CAD build for the part. Positions are in the model's coordinates, mm. Face numbers are marked on the shaded views. A direction names the side the tool comes from. Coordinates: 2 decimals unless noted, no trailing zeros. Loops run counter-clockwise (first coordinate to the right, second up) from the corner with the lowest first, then second, coordinate; pieces in that order, holes last. Notation, with made-up numbers: (60, 43.5) - (85, 43.5) arc R27 cw to (85, 82.5) - close; hole circle Ø5 at (61, 39). An arc over 180 degrees is marked (long way). Put each result on its own line as item: value.
```python
from build123d import *

# Parameters (mm, degrees)
F1_DEPTH = 25.4


with BuildPart() as f1:
    # F0 (on Top) → F1 (new body)
    with BuildSketch(Plane.XY):
        with BuildLine():
            ThreePointArc((0.0883997278, 32.8236170641), (-13.058763384, 37.4885196208), (-20.2230135431, 49.4585962042))
            ThreePointArc((-20.2230135431, 49.4585962042), (-53.4333511512, 0), (-20.2230135431, -49.4585962042))
            ThreePointArc((-20.2230135431, -49.4585962042), (-13.0929285798, -37.5165620637), (0, -32.8234274819))
            Line((0, -32.8234274819), (42.1633208321, -32.8234274819))
            ThreePointArc((42.1633208321, -32.8234274819), (50.5373651023, -17.3521682727), (53.4333511512, 0))
            ThreePointArc((53.4333511512, 0), (50.5373260912, 17.3522818904), (42.1631732449, 32.8236170641))
            Line((42.1631732449, 32.8236170641), (0.0883997278, 32.8236170641))
        make_face()
        with BuildLine():
            ThreePointArc((0, -32.8234274819), (-13.0929285798, -37.5165620637), (-20.2230135431, -49.4585962042))
            ThreePointArc((-20.2230135431, -49.4585962042), (-10.3049618346, -52.4302467745), (0, -53.4333511512))
            ThreePointArc((0, -53.4333511512), (10.3049618346, -52.4302467745), (20.2230135431, -49.4585962042))
            ThreePointArc((20.2230135431, -49.4585962042), (13.0929285798, -37.5165620637), (0, -32.8234274819))
        make_face()
        with BuildLine():
            ThreePointArc((0, -32.8234274819), (13.0929285798, -37.5165620637), (20.2230135431, -49.4585962042))
            ThreePointArc((20.2230135431, -49.4585962042), (32.2830588513, -42.5784819651), (42.1633208321, -32.8234274819))
            Line((42.1633208321, -32.8234274819), (0, -32.8234274819))
        make_face()
        with BuildLine():
            Line((0, -53.4333511512), (20.6099236693, -53.4333511512))
            ThreePointArc((20.6099236693, -53.4333511512), (20.5129680829, -51.436580237), (20.2230135431, -49.4585962042))
            ThreePointArc((20.2230135431, -49.4585962042), (10.3049618346, -52.4302467745), (0, -53.4333511512))
        make_face()
        with BuildLine():
            Line((20.6099236693, -53.4333511512), (51.2570339651, -53.4333511512))
            ThreePointArc((51.2570339651, -53.4333511512), (59.7096740135, -43.7854013954), (66.3703936593, -32.8234274819))
            Line((66.3703936593, -32.8234274819), (42.1633208321, -32.8234274819))
            ThreePointArc((42.1633208321, -32.8234274819), (32.2830588513, -42.5784819651), (20.2230135431, -49.4585962042))
            ThreePointArc((20.2230135431, -49.4585962042), (20.5129680829, -51.436580237), (20.6099236693, -53.4333511512))
        make_face()
        with BuildLine():
            ThreePointArc((102.2053944331, -32.8234274819), (87.6319776468, -38.8599343649), (81.5954707638, -53.4333511512))
            Line((81.5954707638, -53.4333511512), (102.2053944331, -53.4333511512))
            Line((102.2053944331, -53.4333511512), (102.2053944331, -32.8234274819))
        make_face()
        with BuildLine():
            ThreePointArc((20.6099236693, 53.4333511512), (14.5734167863, 68.0067679375), (0, 74.0432748205))
            ThreePointArc((0, 74.0432748205), (-15.9167890876, 66.526279731), (-20.2230135431, 49.4585962042))
            ThreePointArc((-20.2230135431, 49.4585962042), (-10.3049618346, 52.4302467745), (0, 53.4333511512))
            Line((0, 53.4333511512), (20.6099236693, 53.4333511512))
        make_face()
        with BuildLine():
            ThreePointArc((51.2570339651, 53.4333511512), (27.6226921414, 68.6978414873), (0, 74.0432748205))
            ThreePointArc((0, 74.0432748205), (14.5734167863, 68.0067679375), (20.6099236693, 53.4333511512))
            Line((20.6099236693, 53.4333511512), (51.2570339651, 53.4333511512))
        make_face()
        with BuildLine():
            ThreePointArc((81.5954707638, -53.4333511512), (87.6319776468, -68.0067679375), (102.2053944331, -74.0432748205))
            Line((102.2053944331, -74.0432748205), (102.2053944331, -53.4333511512))
            Line((102.2053944331, -53.4333511512), (81.5954707638, -53.4333511512))
        make_face()
        with BuildLine():
            Line((102.2053944331, 74.0432748205), (0, 74.0432748205))
            ThreePointArc((0, 74.0432748205), (27.6226921414, 68.6978414873), (51.2570339651, 53.4333511512))
            Line((51.2570339651, 53.4333511512), (81.5954707638, 53.4333511512))
            ThreePointArc((81.5954707638, 53.4333511512), (87.6319776468, 68.0067679375), (102.2053944331, 74.0432748205))
        make_face()
        with BuildLine():
            ThreePointArc((-20.2230135431, -49.4585962042), (-15.9167890876, -66.526279731), (0, -74.0432748205))
            ThreePointArc((0, -74.0432748205), (14.5734167863, -68.0067679375), (20.6099236693, -53.4333511512))
            Line((20.6099236693, -53.4333511512), (0, -53.4333511512))
            ThreePointArc((0, -53.4333511512), (-10.3049618346, -52.4302467745), (-20.2230135431, -49.4585962042))
        make_face()
        with BuildLine():
            ThreePointArc((122.8153181024, 53.4333511512), (116.7788112194, 68.0067679375), (102.2053944331, 74.0432748205))
            Line((102.2053944331, 74.0432748205), (102.2053944331, 53.4333511512))
            Line((102.2053944331, 53.4333511512), (102.2053944331, 32.8236170641))
            Line((102.2053944331, 32.8236170641), (102.2053944331, 32.8234274819))
            ThreePointArc((102.2053944331, 32.8234274819), (116.7788112194, 38.8599343649), (122.8153181024, 53.4333511512))
        make_face()
        with BuildLine():
            Line((102.2053944331, 53.4333511512), (102.2053944331, 74.0432748205))
            ThreePointArc((102.2053944331, 74.0432748205), (87.6319776468, 68.0067679375), (81.5954707638, 53.4333511512))
            Line((81.5954707638, 53.4333511512), (102.2053944331, 53.4333511512))
        make_face()
        with BuildLine():
            ThreePointArc((20.6099236693, -53.4333511512), (14.5734167863, -68.0067679375), (0, -74.0432748205))
            ThreePointArc((0, -74.0432748205), (27.6226921414, -68.6978414873), (51.2570339651, -53.4333511512))
            Line((51.2570339651, -53.4333511512), (20.6099236693, -53.4333511512))
        make_face()
        with BuildLine():
            ThreePointArc((51.2570339651, -53.4333511512), (27.6226921414, -68.6978414873), (0, -74.0432748205))
            Line((0, -74.0432748205), (102.2053944331, -74.0432748205))
            ThreePointArc((102.2053944331, -74.0432748205), (87.6319776468, -68.0067679375), (81.5954707638, -53.4333511512))
            Line((81.5954707638, -53.4333511512), (51.2570339651, -53.4333511512))
        make_face()
        with BuildLine():
            ThreePointArc((-20.2230135431, 49.4585962042), (-15.9167890876, 66.526279731), (0, 74.0432748205))
            ThreePointArc((0, 74.0432748205), (-74.0432748205, 0), (0, -74.0432748205))
            ThreePointArc((0, -74.0432748205), (-15.9167890876, -66.526279731), (-20.2230135431, -49.4585962042))
            ThreePointArc((-20.2230135431, -49.4585962042), (-53.4333511512, 0), (-20.2230135431, 49.4585962042))
        make_face()
        with BuildLine():
            ThreePointArc((66.3703936593, -32.8234274819), (59.7096740135, -43.7854013954), (51.2570339651, -53.4333511512))
            Line((51.2570339651, -53.4333511512), (81.5954707638, -53.4333511512))
            ThreePointArc((81.5954707638, -53.4333511512), (87.6319776468, -38.8599343649), (102.2053944331, -32.8234274819))
            Line((102.2053944331, -32.8234274819), (66.3703936593, -32.8234274819))
        make_face()
        with BuildLine():
            Line((102.2053944331, 32.8236170641), (102.1169947054, 32.8236170641))
            ThreePointArc((102.1169947054, 32.8236170641), (102.1611944676, 32.8234748775), (102.2053944331, 32.8234274819))
            Line((102.2053944331, 32.8234274819), (102.2053944331, 32.8236170641))
        make_face()
        with BuildLine():
            Line((102.2053944331, -53.4333511512), (102.2053944331, -74.0432748205))
            ThreePointArc((102.2053944331, -74.0432748205), (116.7788112194, -68.0067679375), (122.8153181024, -53.4333511512))
            ThreePointArc((122.8153181024, -53.4333511512), (116.7788112194, -38.8599343649), (102.2053944331, -32.8234274819))
            Line((102.2053944331, -32.8234274819), (102.2053944331, -53.4333511512))
        make_face()
        with BuildLine():
            Line((102.2053944331, 53.4333511512), (81.5954707638, 53.4333511512))
            ThreePointArc((81.5954707638, 53.4333511512), (87.6007570653, 38.891221974), (102.1169947054, 32.8236170641))
            Line((102.1169947054, 32.8236170641), (102.2053944331, 32.8236170641))
            Line((102.2053944331, 32.8236170641), (102.2053944331, 53.4333511512))
        make_face()
        with BuildLine():
            Line((81.5954707638, 53.4333511512), (51.2570339651, 53.4333511512))
            ThreePointArc((51.2570339651, 53.4333511512), (59.7096114785, 43.7854866736), (66.3702999012, 32.8236170641))
            Line((66.3702999012, 32.8236170641), (102.1169947054, 32.8236170641))
            ThreePointArc((102.1169947054, 32.8236170641), (87.6007570653, 38.891221974), (81.5954707638, 53.4333511512))
        make_face()
        with BuildLine():
            ThreePointArc((66.3702999012, 32.8236170641), (59.7096114785, 43.7854866736), (51.2570339651, 53.4333511512))
            Line((51.2570339651, 53.4333511512), (20.6099236693, 53.4333511512))
            ThreePointArc((20.6099236693, 53.4333511512), (20.5129680829, 51.436580237), (20.2230135431, 49.4585962042))
            ThreePointArc((20.2230135431, 49.4585962042), (32.2829631266, 42.5785545435), (42.1631732449, 32.8236170641))
            Line((42.1631732449, 32.8236170641), (66.3702999012, 32.8236170641))
        make_face()
        with BuildLine():
            ThreePointArc((20.2230135431, 49.4585962042), (20.5129680829, 51.436580237), (20.6099236693, 53.4333511512))
            Line((20.6099236693, 53.4333511512), (0, 53.4333511512))
            ThreePointArc((0, 53.4333511512), (10.3049618346, 52.4302467745), (20.2230135431, 49.4585962042))
        make_face()
        with BuildLine():
            ThreePointArc((0, 53.4333511512), (-10.3049618346, 52.4302467745), (-20.2230135431, 49.4585962042))
            ThreePointArc((-20.2230135431, 49.4585962042), (-13.058763384, 37.4885196208), (0.0883997278, 32.8236170641))
            ThreePointArc((0.0883997278, 32.8236170641), (13.1270335572, 37.5446777126), (20.2230135431, 49.4585962042))
            ThreePointArc((20.2230135431, 49.4585962042), (10.3049618346, 52.4302467745), (0, 53.4333511512))
        make_face()
        with BuildLine():
            ThreePointArc((74.0432748205, 0), (72.0995176879, 16.8542604501), (66.3702999012, 32.8236170641))
            Line((66.3702999012, 32.8236170641), (42.1631732449, 32.8236170641))
            ThreePointArc((42.1631732449, 32.8236170641), (50.5373260912, 17.3522818904), (53.4333511512, 0))
            Line((53.4333511512, 0), (74.0432748205, 0))
        make_face()
        with BuildLine():
            Line((42.1633208321, -32.8234274819), (66.3703936593, -32.8234274819))
            ThreePointArc((66.3703936593, -32.8234274819), (72.0995417593, -16.8541574765), (74.0432748205, 0))
            Line((74.0432748205, 0), (53.4333511512, 0))
            ThreePointArc((53.4333511512, 0), (50.5373651023, -17.3521682727), (42.1633208321, -32.8234274819))
        make_face()
        with BuildLine():
            ThreePointArc((42.1631732449, 32.8236170641), (32.2829631266, 42.5785545435), (20.2230135431, 49.4585962042))
            ThreePointArc((20.2230135431, 49.4585962042), (13.1270335572, 37.5446777126), (0.0883997278, 32.8236170641))
            Line((0.0883997278, 32.8236170641), (42.1631732449, 32.8236170641))
        make_face()
    extrude(amount=F1_DEPTH)


solid = f1.part
```
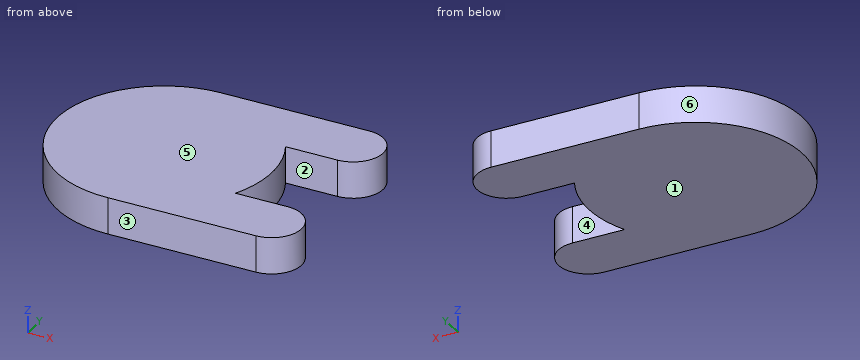
Q1. Slice it at D-D, the plane x = -34. Give the cut face in (y, z), then the cut area to 3 significant figures.
Determined:
outline: (-65.78, 0) - (65.78, 0) - (65.78, 25.4) - (-65.78, 25.4) - close
area: 3,340 mm2
Q2. Slice it at A-A, the plane z = 2. Give the cut face in (x, y).
Determined:
outline: (0, -74.04) - (102.21, -74.04) arc R20.61 ccw to (102.21, -32.82) - (66.37, -32.82) arc R74.04 ccw to (66.37, 32.82) - (102.12, 32.82) arc R20.61 ccw to (102.21, 32.82) arc R20.61 ccw to (102.21, 74.04) - (0, 74.04) arc R74.04 ccw to start
Q3. Slice it at B-B, the plane x = 71. Give the cut face in (y, z).
Determined:
outline: (-74.04, 0) - (-32.82, 0) - (-32.82, 25.4) - (-74.04, 25.4) - close; (-21.01, 0) - (21.01, 0) - (21.01, 25.4) - (-21.01, 25.4) - close; (32.82, 0) - (74.04, 0) - (74.04, 25.4) - (32.82, 25.4) - close
Q4. Slice it at C-C, the plane y = 0. Give the cut face in (x, z).
Determined:
outline: (-74.04, 0) - (74.04, 0) - (74.04, 25.4) - (-74.04, 25.4) - close
Q5. Wall check: L1, parallel to Y at x = 96, z = 20; L2, parallel to X at y = -4, z = 8.5; L3, parallel to X at y = -15, z = 14.5. Give the ranges that are in metal, low to high. Write a range as from..to.
Determined:
L1: -74.04..-32.82, 32.82..74.04
L2: -73.94..73.94
L3: -72.51..72.51
Q6. Pin check, flat tips, straight feed: pin 1 Ø6 at (x, z) = (-7, 13) entering from -Y; pin 2 Ø8 at (x, z) = (-41, 5) entering from +Y; pin 3 Ø1 at (y, z) = (1, 4.5) entering from -X. Stop position of each tip, or through.
Determined:
pin 1: y = -73.94
pin 2: y = 64.14
pin 3: x = -74.04
Q7. Tool access for the marked faces 1 and 2: list every direction of +Z, -Z, +X, -X, +Y, -Y with a clear straight run to the whole face (end or side of a thin tool).
Determined:
face 1: -Z, +X, -X, +Y, -Y
face 2: +Z, -Z, +X
Q8. Mould opens along Y. For the marked faces 3, 4, 5 and 6 say: +Y half, -Y half, draft (parallel to the pull), parting line (faces both ways), or undercut.
Determined:
face 3: -Y half
face 4: undercut
face 5: draft
face 6: parting line
